from build123d import *

# Parameters (mm, degrees)
EXTRUDE_1_DEPTH = 47


with BuildPart() as part:
    # 草图1 → 凸台-拉伸1 (new body)
    with BuildSketch(Plane.XY):
        with BuildLine():
            Line((18.639450369, 45.736574885), (46.639450369, 45.736574885))
            ThreePointArc((46.639450369, 45.736574885), (47.34655715, 45.443681666), (47.639450369, 44.736574885))
            Line((47.639450369, 44.736574885), (47.639450369, -153.263425115))
            ThreePointArc((47.639450369, -153.263425115), (47.34655715, -153.970531897), (46.639450369, -154.263425115))
            Line((46.639450369, -154.263425115), (-262.360549631, -154.263425115))
            ThreePointArc((-262.360549631, -154.263425115), (-263.067656412, -153.970531897), (-263.360549631, -153.263425115))
            Line((-263.360549631, -153.263425115), (-263.360549631, 44.736574885))
            ThreePointArc((-263.360549631, 44.736574885), (-263.067656412, 45.443681666), (-262.360549631, 45.736574885))
            Line((-262.360549631, 45.736574885), (-234.360549631, 45.736574885))
            ThreePointArc((-234.360549631, 45.736574885), (-233.65344285, 45.443681666), (-233.360549631, 44.736574885))
            Line((-233.360549631, 44.736574885), (-233.360549631, 33.736574885))
            ThreePointArc((-233.360549631, 33.736574885), (-233.067656412, 33.029468103), (-232.360549631, 32.736574885))
            Line((-232.360549631, 32.736574885), (-223.360549631, 32.736574885))
            Line((-223.360549631, 32.736574885), (-223.360549631, 34.236574885))
            Line((-223.360549631, 34.236574885), (-230.860549631, 34.236574885))
            ThreePointArc((-230.860549631, 34.236574885), (-231.567656412, 34.529468103), (-231.860549631, 35.236574885))
            Line((-231.860549631, 35.236574885), (-231.860549631, 46.236574885))
            ThreePointArc((-231.860549631, 46.236574885), (-232.15344285, 46.943681666), (-232.860549631, 47.236574885))
            Line((-232.860549631, 47.236574885), (-263.860549631, 47.236574885))
            ThreePointArc((-263.860549631, 47.236574885), (-264.567656412, 46.943681666), (-264.860549631, 46.236574885))
            Line((-264.860549631, 46.236574885), (-264.860549631, -154.763425115))
            ThreePointArc((-264.860549631, -154.763425115), (-264.567656412, -155.470531897), (-263.860549631, -155.763425115))
            Line((-263.860549631, -155.763425115), (48.139450369, -155.763425115))
            ThreePointArc((48.139450369, -155.763425115), (48.84655715, -155.470531897), (49.139450369, -154.763425115))
            Line((49.139450369, -154.763425115), (49.139450369, 46.236574885))
            ThreePointArc((49.139450369, 46.236574885), (48.84655715, 46.943681666), (48.139450369, 47.236574885))
            Line((48.139450369, 47.236574885), (17.139450369, 47.236574885))
            ThreePointArc((17.139450369, 47.236574885), (16.432343588, 46.943681666), (16.139450369, 46.236574885))
            Line((16.139450369, 46.236574885), (16.139450369, 35.236574885))
            ThreePointArc((16.139450369, 35.236574885), (15.84655715, 34.529468103), (15.139450369, 34.236574885))
            Line((15.139450369, 34.236574885), (7.639450369, 34.236574885))
            Line((7.639450369, 34.236574885), (7.639450369, 32.736574885))
            Line((7.639450369, 32.736574885), (16.639450369, 32.736574885))
            ThreePointArc((16.639450369, 32.736574885), (17.34655715, 33.029468103), (17.639450369, 33.736574885))
            Line((17.639450369, 33.736574885), (17.639450369, 44.736574885))
            ThreePointArc((17.639450369, 44.736574885), (17.932343588, 45.443681666), (18.639450369, 45.736574885))
        make_face()
    extrude(amount=EXTRUDE_1_DEPTH)


solid = part.part
Verification items for the finished model (mm, model axes). A direction names the side the tool comes from. Give positions to 0.01 mm unless a question says otherwise; leave off trailing zeros. Write each loop counter-clockwise with the first axis right and the second up, starting at its lowest first coordinate (ties: lowest second). Pieces come first, ordered by that corner, then holes.
(1) Cross-section at A-A (y = -74). Enter the section's corners in (x, z).
(2) Material ranges on line 1 (X direction, y = 0, z = 43); line 2 (Y direction, x = -224, z = 13); line 3 (Y direction, x = 23, z = 10.5), recorded low to high.
(3) Mould release check, pull along X, two halves, no side actions. Record for faces 1 (the face through (49.139, -56, 23)), 2 (the face through (33, 47.237, 23)), 3 (the face through (-249, 45.737, 23)): +X half, -X half, draft (parallel to the pull), parting line (faces both ways), or undercut.
(4) Gauge pin test, flat ends, axial feed: pin 1 (8 mm diameter, centred on x = 9.5, z = 30, fed in from +Y); pin 2 (4 mm diameter, centred on x = -63.5, z = 6.5, fed in from +Y). Record the tip position at first contact, or that the pin passes through.
(5) Cross-section at B-B (x = -43.5). Enter the section's corners in (y, z).
(6) Access from +Z, -Z, +X, -X, +Y, -Y to the whole of each face (thin tool, end or side, straight path). Record for faces 4 (the face through (-110, -155.763, 23)), 5 (the face through (11, 34.237, 23)), 6 (the face through (12, 32.737, 23)).
Worked out:
1. outline: (-264.86, 0) - (-263.36, 0) - (-263.36, 47) - (-264.86, 47) - close; (47.64, 0) - (49.14, 0) - (49.14, 47) - (47.64, 47) - close
2. line 1: x = -264.86 to -263.36, 47.64 to 49.14
2. line 2: y = -155.76 to -154.26, 32.74 to 34.24
2. line 3: y = -155.76 to -154.26, 45.74 to 47.24
3. face 1: +X half
3. face 2: draft
3. face 3: undercut
4. pin 1: stops at y = 34.24
4. pin 2: stops at y = -154.26
5. outline: (-155.76, 0) - (-154.26, 0) - (-154.26, 47) - (-155.76, 47) - close
6. face 4: +Z, -Z, +X, -X, -Y
6. face 5: +Z, -Z, +Y
6. face 6: +Z, -Z
